from build123d import *

# Parameters (mm, degrees)
CHAMFER_1_SIZE  = 0.8
CHAMFER_1_SIZE2 = 0.214359354
CHAMFER_2_SIZE  = 1.2


with BuildPart() as part:
    # Эскиз3 → Повернуть1 (revolve)
    with BuildSketch(Plane.XY):
        Polygon((-4, 0), (-9, 0), (-9, 3), (-7, 3), (-7, 10), (-4, 10), align=None)
    revolve(axis=Axis((0, -11.687612648, 0), (0, 1, 0)))

    # Фаска1
    chamfer_1_edges = [part.edges().sort_by_distance(p)[0] for p in [
        (7, 10, 0),
    ]]
    chamfer_1_side = [part.faces().sort_by_distance(p)[0] for p in [
        (6.802010101, 10, 0),
    ]]
    chamfer(chamfer_1_edges, length=CHAMFER_1_SIZE, length2=CHAMFER_1_SIZE2, reference=chamfer_1_side[0])

    # Фаска2
    chamfer_2_edges = [part.edges().sort_by_distance(p)[0] for p in [
        (4, 10, 0),
    ]]
    chamfer(chamfer_2_edges, length=CHAMFER_2_SIZE)


solid = part.part
For this review, take the finished solid that the model builds, in its own axes (mm). A direction names the side the tool comes from. Give positions to 0.01 mm unless a question says otherwise; leave off trailing zeros. Order: outer loops, then holes, each group sorted by start corner. A loop starts at its lowest first (then second) coordinate and runs counter-clockwise, first axis right, second up. Notation, with made-up numbers: (76, 67) -> (84, 67) arc R24 ccw to (84, 96) -> close; hole circle Ø10 at (-11.75, 83.25). An arc over 180 degrees is marked (long way). Write item = value, one per line.
1) We need section B-B, the plane x = 0. Give the boundary of the cut face in (y, z).
Findings:
outline = (0, -9) -> (3, -9) -> (3, -7) -> (9.79, -7) -> (10, -6.2) -> (10, -5.2) -> (8.8, -4) -> (0, -4) -> close; (0, 4) -> (8.8, 4) -> (10, 5.2) -> (10, 6.2) -> (9.79, 7) -> (3, 7) -> (3, 9) -> (0, 9) -> close
2) We need section D-D, the plane y = 6. Give the boundary of the cut face in (x, z).
Findings:
outline = circle Ø14 at (0, 0); hole circle Ø8 at (0, 0)
3) We need section C-C, the plane y = 2.25. Give the boundary of the cut face in (x, z).
Findings:
outline = circle Ø18 at (0, 0); hole circle Ø8 at (0, 0)
4) Insertion check: pin 1 (9 mm diameter, centred on x = 0, z = 0, fed in from +Y); pin 2 (4 mm diameter, centred on x = -5, y = 8, fed in from -Z); pin 3 (5 mm diameter, centred on y = 7, z = -2, fed in from +X). Each pin has a flat end and moves straight along its axis. Give the tip position at first contact, or say it passes through.
Findings:
pin_1 = 9.3
pin_2 = -6.32
pin_3 = 7
5) Draft analysis for pull direction Z (two halves, no side actions). For faces 3 (the face through (0.867, 4.338, -3.905)), 4 (the face through (2, 0, -4)), 5 (the face through (-6.466, 6.44, -2.681)), state which applies: pulls with the +Z half, pulls with the -Z half, needs draft (parallel to the pull), parting line crosses it, or undercut.
Findings:
face_3 = undercut
face_4 = needs draft
face_5 = parting line crosses it
6) We need section A-A, the plane z = 0. Give the boundary of the cut face in (x, y).
Findings:
outline = (-9, 0) -> (-4, 0) -> (-4, 8.8) -> (-5.2, 10) -> (-6.2, 10) -> (-7, 9.79) -> (-7, 3) -> (-9, 3) -> close; (4, 0) -> (9, 0) -> (9, 3) -> (7, 3) -> (7, 9.79) -> (6.2, 10) -> (5.2, 10) -> (4, 8.8) -> close
7) For faces 1 (the face through (0, 3, -7.3)), 2 (the face through (1.172, 1.521, 8.923)), list the 3-axis set-ups (+Z, -Z, +X, -X, +Y, -Y) from which the entire face can be reached by the end or side of a thin tool; tool diameter is ignored.
Findings:
face_1 = +Y
face_2 = +Y, -Y
8) To check wall thickness, follow L1, parallel to Z at x = 0, y = 3.5; L2, parallel to Z at x = 0, y = 2; L3, parallel to X at y = 3.5, z = -2.75. State the ranges of each line that lie inside material, in increasing order. Write a range as from..to.
Findings:
L1 = -7..-4, 4..7
L2 = -9..-4, 4..9
L3 = -6.44..-2.9, 2.9..6.44
